```python
from build123d import *

# Parameters (mm, degrees)
SKETCH1_R                   = 5
BOSS_EXTRUDE1_DEPTH         = 1.5
SKETCH2_R                   = 10.85
BOSS_EXTRUDE2_DEPTH         = 3.4
SKETCH3_R                   = 4.95
BOSS_EXTRUDE3_DEPTH         = 9.8
M8_TAPPED_HOLE1_D           = 6.8
M8_TAPPED_HOLE1_CSINK_D     = 8.05
M8_TAPPED_HOLE1_CSINK_ANGLE = 90
SKETCH6_R                   = 1.75
CUT_EXTRUDE1_DEPTH          = 21.240676866


with BuildPart() as part:
    # Sketch1 → Boss-Extrude1 (new body)
    with BuildSketch(Plane(origin=(0, 0, 0), x_dir=(1, 0, 0), z_dir=(0, 1, 0))):
        with Locations(Location((0, 0, 0), (0, 0, 270))):
            Circle(SKETCH1_R)
    extrude(amount=BOSS_EXTRUDE1_DEPTH)

    # Sketch2 → Boss-Extrude2 (add)
    with BuildSketch(Plane(origin=(0, 1.5, 0), x_dir=(1, 0, 0), z_dir=(0, 1, 0))):
        with Locations(Location((0, 0, 0), (0, 0, 270))):
            Circle(SKETCH2_R)
    extrude(amount=BOSS_EXTRUDE2_DEPTH)

    # Sketch3 → Boss-Extrude3 (add)
    with BuildSketch(Plane(origin=(0, 4.9, 0), x_dir=(1, 0, 0), z_dir=(0, 1, 0))):
        with Locations(Location((0, 0, 0), (0, 0, 270))):
            Circle(SKETCH3_R)
    extrude(amount=BOSS_EXTRUDE3_DEPTH)

    # M8 Tapped Hole1 (through all)
    with Locations(Plane(origin=(0, 0, 0), x_dir=(0, 0, -1), z_dir=(0, -1, 0))):
        with Locations((0, 0)):
            CounterSinkHole(M8_TAPPED_HOLE1_D / 2, M8_TAPPED_HOLE1_CSINK_D / 2, counter_sink_angle=M8_TAPPED_HOLE1_CSINK_ANGLE)

    # Sketch6 → Cut-Extrude1 (cut, through all)
    with BuildSketch(Plane.XZ.offset(-1.5)):
        with Locations(Location((-0.016416422, 8.449812512, 0), (0, 0, 270))):
            Circle(SKETCH6_R)
        with Locations(Location((8.449812512, 0.016416422, 0), (0, 0, 270))):
            Circle(SKETCH6_R)
        with Locations(Location((0.016416422, -8.449812512, 0), (0, 0, 270))):
            Circle(SKETCH6_R)
        with Locations(Location((-8.449812512, -0.016416422, 0), (0, 0, 270))):
            Circle(SKETCH6_R)
    extrude(amount=-CUT_EXTRUDE1_DEPTH, mode=Mode.SUBTRACT)


solid = part.part
```
Verification items for the finished model (mm, model axes). A direction names the side the tool comes from. Coordinates: 2 decimals unless noted, no trailing zeros. Write each loop counter-clockwise with the first axis right and the second up, starting at its lowest first coordinate (ties: lowest second). Pieces come first, ordered by that corner, then holes. Notation, with made-up numbers: M -1.5,48.25 L 35.5,48.25 A14 ccw 35.5,73.25 Z; hole C -14,-28.5 d9. An arc over 180 degrees is marked long. One line per item, written item: value.
Item 1: Access from +Z, -Z, +X, -X, +Y, -Y to the whole of each face (thin tool, end or side, straight path). Record for faces 4 (the cylindrical face through (-4.88, 0.74, -1.08)), 5 (the cylindrical face through (-1.7, 3.2, -8.1)), 6 (the flat face through (-2, 4.9, 5)).
Check sheet entries:
face 4: -Y
face 5: +Y, -Y
face 6: +Y
Item 2: Mould release check, pull along Z, two halves, no side actions. Record for faces 1 (the cylindrical face through (3.26, 3.18, 10.35)), 2 (the cylindrical face through (10.185, 3.176, 0.244)), 3 (the flat face through (-2, 1.5, 5)): pulls with the +Z half, pulls with the -Z half, needs draft (parallel to the pull), parting line crosses it, or undercut.
Check sheet entries:
face 1: parting line crosses it
face 2: undercut
face 3: needs draft
Item 3: Section check A-A, the plane z = -7.75. Record the boundary of the cut face in (x, y).
Check sheet entries:
outline: M -7.59,1.5 L -1.59,1.5 L -1.59,4.9 L -7.59,4.9 Z; M 1.62,1.5 L 7.59,1.5 L 7.59,4.9 L 1.62,4.9 Z
Item 4: Scan lines: line 1 along X through (y, z) = (4.5, 0); line 2 along Z through (x, y) = (-1.5, 3.75); line 3 along Y through (x, z) = (-5, 6). Record each from-to range of solid material in increasing order.
Check sheet entries:
line 1: x = -10.85 to -10.2, -6.7 to -3.4, 3.4 to 6.7, 10.2 to 10.85
line 2: z = -10.75 to -9.32, -7.58 to -3.05, 3.05 to 7.52, 9.38 to 10.75
line 3: y = 1.5 to 4.9
Item 5: Section check D-D, the plane y = 12.5. Record the boundary of the cut face in (x, z).
Check sheet entries:
outline: C 0,0 d9.9; hole C 0,0 d6.8
Item 6: Section check C-C, the plane z = 0. Record the boundary of the cut face in (x, y) (3 decimals), plus the area to 3 significant figures.
Check sheet entries:
outline: M -10.85,1.5 L -10.2,1.5 L -10.2,4.9 L -10.85,4.9 Z; M -6.7,1.5 L -5,1.5 L -5,0 L -4.025,0 L -3.4,0.625 L -3.4,14.7 L -4.95,14.7 L -4.95,4.9 L -6.7,4.9 Z; M 3.4,0.625 L 4.025,0 L 5,0 L 5,1.5 L 6.7,1.5 L 6.7,4.9 L 4.95,4.9 L 4.95,14.7 L 3.4,14.7 Z; M 10.2,1.5 L 10.85,1.5 L 10.85,4.9 L 10.2,4.9 Z
area: 61.7 mm^2
Item 7: Gauge pin test, flat ends, axial feed: pin 1 Ø3 at (x, z) = (-8.45, -0.02) entering from -Y; pin 2 Ø1 at (x, y) = (8.5, 4.5) entering from +Z; pin 3 Ø6 at (x, y) = (4, 9.5) entering from +Z; pin 4 Ø5.5 at (x, z) = (0.02, -8.45) entering from +Y. Record the tip position at first contact, or that the pin passes through.
Check sheet entries:
pin 1: passes through
pin 2: stops at z = 7.33
pin 3: stops at z = 4.85
pin 4: stops at y = 4.9
Item 8: Section check B-B, the plane x = -8. Record the boundary of the cut face in (y, z), plus the area to 3 significant figures.
Check sheet entries:
outline: M 1.5,-7.33 L 4.9,-7.33 L 4.9,-1.71 L 1.5,-1.71 Z; M 1.5,1.67 L 4.9,1.67 L 4.9,7.33 L 1.5,7.33 Z
area: 38.3 mm^2
